Source: CAD feature listing. Evaluate the final solid. Frame: model axes, mm. A direction names the side the tool comes from. Give positions to 0.01 mm unless a question says otherwise; leave off trailing zeros. Order: outer loops, then holes, each group sorted by start corner. A loop starts at its lowest first (then second) coordinate and runs counter-clockwise, first axis right, second up. Notation, with made-up numbers: (62.5, 17.5) -> (103.5, 17.5) arc R21 ccw to (103.5, 56.5) -> close; hole circle Ø8 at (48.25, 39.25). An arc over 180 degrees is marked (long way). Answer in a Markdown table with one row per item.
Autodesk Inventor part; units mm, degrees
ref_plane "YZ Plane" through (0, 0, 0) normal (1, 0, 0) x (0, 1, 0)
ref_plane "XZ Plane" through (0, 0, 0) normal (0, 1, 0) x (-1, 0, 0)
ref_plane "XY Plane" through (0, 0, 0) normal (0, 0, 1) x (1, 0, 0)
sketch "Sketch1" plane through (0, 0, 0) normal (0, 1, 0) x (-1, 0, 0)
  line L0 (0, 0) -> (20, 0)
  line L1 (20, 0) -> (20, -196.3)
  line L2 (20, -196.3) -> (0, -196.3)
  line L3 (0, -196.3) -> (0, 0)
  dimension "d0" = 20
  dimension "d1" = 196.3
extrude "Extrusion1" add sketch "Sketch1" along normal blind 4
sketch "Sketch2" plane through (0, 4, 0) normal (0, 1, 0) x (1, 0, 0)
  line L0 (-20, 0) -> (0, 0)
  line L1 (0, 0) -> (0, 196.3)
  line L2 (-20, 0) -> (0, 0)
  line L3 (0, 0) -> (0, 8)
  line L4 (0, 8) -> (-20, 8)
  line L5 (-20, 8) -> (-20, 0)
  line L6 (-20, 8) -> (0, 8)
  line L7 (0, 8) -> (0, 48.3)
  line L8 (0, 48.3) -> (-20, 48.3)
  line L9 (-20, 48.3) -> (-20, 8)
  line L10 (-20, 48.3) -> (0, 48.3)
  line L11 (0, 48.3) -> (0, 56.3)
  line L12 (0, 56.3) -> (-20, 56.3)
  line L13 (-20, 56.3) -> (-20, 48.3)
  line L14 (-20, 196.3) -> (-20, 0)
  line L15 (-20, 196.3) -> (0, 196.3)
  line L16 (0, 196.3) -> (0, 188.3)
  line L17 (0, 188.3) -> (-20, 188.3)
  line L18 (-20, 188.3) -> (-20, 196.3)
  line L19 (-20, 188.3) -> (0, 188.3)
  line L20 (0, 188.3) -> (0, 148)
  line L21 (0, 148) -> (-20, 148)
  line L22 (-20, 148) -> (-20, 188.3)
  line L23 (-20, 148) -> (0, 148)
  line L24 (0, 148) -> (0, 140)
  line L25 (0, 140) -> (-20, 140)
  line L26 (-20, 140) -> (-20, 148)
  line L27 (-20, 0) -> (-15, 0)
  line L28 (-15, 0) -> (-15, 8)
  line L29 (-15, 8) -> (-20, 8)
  line L30 (-20, 8) -> (-20, 0)
  line L31 (0, 8) -> (-5, 8)
  line L32 (-5, 8) -> (-5, 0)
  line L33 (-5, 0) -> (0, 0)
  line L34 (0, 0) -> (0, 8)
  line L35 (-20, 48.3) -> (-15, 48.3)
  line L36 (-15, 48.3) -> (-15, 56.3)
  line L37 (-15, 56.3) -> (-20, 56.3)
  line L38 (-20, 56.3) -> (-20, 48.3)
  line L39 (0, 48.3) -> (-5, 48.3)
  line L40 (-5, 48.3) -> (-5, 56.3)
  line L41 (-5, 56.3) -> (0, 56.3)
  line L42 (0, 56.3) -> (0, 48.3)
  line L43 (-20, 140) -> (-15, 140)
  line L44 (-15, 140) -> (-15, 148)
  line L45 (-15, 148) -> (-20, 148)
  line L46 (-20, 148) -> (-20, 140)
  line L47 (0, 140) -> (-5, 140)
  line L48 (-5, 140) -> (-5, 148)
  line L49 (-5, 148) -> (0, 148)
  line L50 (0, 148) -> (0, 140)
  line L51 (-20, 188.3) -> (-15, 188.3)
  line L52 (-15, 188.3) -> (-15, 196.3)
  line L53 (-15, 196.3) -> (-20, 196.3)
  line L54 (-20, 196.3) -> (-20, 188.3)
  line L55 (0, 188.3) -> (-5, 188.3)
  line L56 (-5, 188.3) -> (-5, 196.3)
  line L57 (-5, 196.3) -> (0, 196.3)
  line L58 (0, 196.3) -> (0, 188.3)
  point P0 (0, 188.3)
  point P1 (-15, 140)
  point P2 (-20, 148)
  point P3 (-20, 140)
  dimension "d4" = 8
  dimension "d5" = 40.3
  dimension "d6" = 8
  dimension "d7" = 20
  dimension "d8" = 8
  dimension "d9" = 40.3
  dimension "d10" = 8
  dimension "d11" = 5
  dimension "d12" = 5
  dimension "d13" = 8
  dimension "d14" = 5
  dimension "d15" = 5
  dimension "d16" = 5
  dimension "d17" = 5
  dimension "d18" = 5
  dimension "d19" = 5
extrude "Extrusion2" add sketch "Sketch2" along normal blind 10 contours L5 L4 L28 L0 | L32 L4 L1 L0 | L13 L12 L36 L8 | L40 L12 L1 L8 | L14 L21 L44 L25 | L14 L15 L52 L17 | L48 L21 L1 L25 | L56 L15 L1 L17
sketch "Sketch3" plane through (0, 14, 0) normal (0, 1, 0) x (1, 0, 0)
  line L0 (-20, 196.3) -> (-20, 0)
  line L1 (-20, 0) -> (-17.5, 0)
  line L2 (-17.5, 0) -> (-17.5, 4)
  line L3 (-17.5, 4) -> (-20, 4)
  line L4 (-20, 4) -> (-20, 0)
  line L5 (0, 0) -> (0, 196.3)
  line L6 (0, 0) -> (-2.5, 0)
  line L7 (-2.5, 0) -> (-2.5, 4)
  line L8 (-2.5, 4) -> (0, 4)
  line L9 (0, 4) -> (0, 0)
  line L10 (-15, 56.3) -> (-20, 56.3)
  line L11 (-20, 56.3) -> (-17.5, 56.3)
  line L12 (-17.5, 56.3) -> (-17.5, 52.3)
  line L13 (-17.5, 52.3) -> (-20, 52.3)
  line L14 (-20, 52.3) -> (-20, 56.3)
  line L15 (-5, 56.3) -> (0, 56.3)
  line L16 (-5, 56.3) -> (-2.5, 56.3)
  line L17 (-2.5, 56.3) -> (-2.5, 52.3)
  line L18 (-2.5, 52.3) -> (-5, 52.3)
  line L19 (-5, 52.3) -> (-5, 56.3)
  line L20 (-20, 196.3) -> (-17.5, 196.3)
  line L21 (-17.5, 196.3) -> (-17.5, 192.3)
  line L22 (-17.5, 192.3) -> (-20, 192.3)
  line L23 (-20, 192.3) -> (-20, 196.3)
  line L24 (-5, 196.3) -> (-2.5, 196.3)
  line L25 (-2.5, 196.3) -> (-2.5, 192.3)
  line L26 (-2.5, 192.3) -> (-5, 192.3)
  line L27 (-5, 192.3) -> (-5, 196.3)
  line L28 (-20, 148) -> (-15, 148)
  line L29 (-15, 148) -> (-17.5, 148)
  line L30 (-17.5, 148) -> (-17.5, 144)
  line L31 (-17.5, 144) -> (-15, 144)
  line L32 (-15, 144) -> (-15, 148)
  line L33 (-5, 148) -> (-2.5, 148)
  line L34 (-2.5, 148) -> (-2.5, 144)
  line L35 (-2.5, 144) -> (-5, 144)
  line L36 (-5, 144) -> (-5, 148)
  circle A0 centre (-17.5, 144) radius 1.5
  circle A1 centre (-2.5, 144) radius 1.5
  circle A2 centre (-17.5, 192.3) radius 1.5
  circle A3 centre (-2.5, 192.3) radius 1.5
  circle A4 centre (-17.5, 52.3) radius 1.5
  circle A5 centre (-2.5, 52.3) radius 1.5
  circle A6 centre (-17.5, 4) radius 1.5
  circle A7 centre (-2.5, 4) radius 1.5
  dimension "d22" = 2.5
  dimension "d23" = 4
  dimension "d24" = 2.5
  dimension "d25" = 4
  dimension "d26" = 2.5
  dimension "d27" = 4
  dimension "d28" = 2.5
  dimension "d29" = 4
  dimension "d30" = 2.5
  dimension "d31" = 4
  dimension "d32" = 2.5
  dimension "d33" = 4
  dimension "d34" = 2.5
  dimension "d35" = 4
  dimension "d36" = 2.5
  dimension "d37" = 4
  dimension "d38" = 3
  dimension "d39" = 3
  dimension "d40" = 3
  dimension "d41" = 3
  dimension "d42" = 3
  dimension "d43" = 3
  dimension "d44" = 3
  dimension "d45" = 3
extrude "Extrusion3" cut sketch "Sketch3" against normal up to surface (14 mm away) contours A2 L21 L22 | L22 L21 A2 | A0 L31 L30 | L30 L31 A0 | A4 L12 L13 | L13 L12 A4 | A6 L2 L3 | L3 L2 A6 | A7 L7 L8 | L8 L7 A7 | A5 L18 L17 | L17 L18 A5 | A3 L26 L25 | L25 L26 A3 | A1 L35 L34 | L34 L35 A1
fillet "Fillet1" radius 3 12 edges at (-15, 4, -52.3) (-5, 4, -52.3) (-15, 4, -144) (-2.5, 4, -140) (-2.5, 4, -56.3) (-5, 4, -144) (-15, 4, -4) (-5, 4, -4) (-15, 4, -192.3) (-5, 4, -192.3) (-17.5, 4, -56.3) (-17.5, 4, -140)
sketch "Sketch5" plane through (0, 4, 0) normal (0, 1, 0) x (1, 0, 0)
  line L0 (0, 48.3) -> (-8, 48.3)
  line L1 (0, 48.3) -> (-4, 48.3)
  line L2 (-8, 148) -> (0, 148)
  line L3 (0, 148) -> (-4, 148)
  line L4 (-4, 148) -> (-16, 148)
  line L5 (-16, 148) -> (-16, 168)
  line L6 (-16, 168) -> (-4, 168)
  line L7 (-4, 168) -> (-4, 148)
  line L8 (-4, 48.3) -> (-16, 48.3)
  line L9 (-16, 48.3) -> (-16, 28.3)
  line L10 (-16, 28.3) -> (-4, 28.3)
  line L11 (-4, 28.3) -> (-4, 48.3)
  point P0 (0, 0)
  dimension "d63" = 4
  dimension "d64" = 4
  dimension "d65" = 12
  dimension "d66" = 20
  dimension "d67" = 12
  dimension "d68" = 20
extrude "Extrusion5" cut sketch "Sketch5" against normal blind 8
sketch "Sketch6" plane through (0, 0, 0) normal (0, -1, 0) x (1, 0, 0)
  circle A0 centre (-2.5, -4) radius 1.5
  circle A1 centre (-2.5, -4) radius 4
  circle A2 centre (-17.5, -4) radius 1.5
  circle A3 centre (-17.5, -4) radius 4
  circle A4 centre (-17.5, -52.3) radius 1.5
  circle A5 centre (-17.5, -52.3) radius 4
  circle A6 centre (-2.5, -52.3) radius 1.5
  circle A7 centre (-2.5, -52.3) radius 4
  circle A8 centre (-17.5, -144) radius 1.5
  circle A9 centre (-17.5, -144) radius 4
  circle A10 centre (-2.5, -144) radius 1.5
  circle A11 centre (-2.5, -144) radius 4
  circle A12 centre (-17.5, -192.3) radius 1.5
  circle A13 centre (-17.5, -192.3) radius 4
  circle A14 centre (-2.5, -192.3) radius 1.5
  circle A15 centre (-2.5, -192.3) radius 4
  line L0 (0, -196.3) -> (-20, -196.3)
  line L1 (-20, -196.3) -> (-17.5, -196.3)
  line L2 (-17.5, -196.3) -> (-17.5, -192.3)
  line L3 (-17.5, -192.3) -> (-20, -192.3)
  line L4 (-20, -192.3) -> (-20, -196.3)
  line L5 (0, -196.3) -> (-2.5, -196.3)
  line L6 (-2.5, -196.3) -> (-2.5, -192.3)
  line L7 (-2.5, -192.3) -> (0, -192.3)
  line L8 (0, -192.3) -> (0, -196.3)
  line L9 (-20, -196.3) -> (-20, 0)
  line L10 (-20, 0) -> (-17.5, 0)
  line L11 (-17.5, 0) -> (-17.5, -4)
  line L12 (-17.5, -4) -> (-20, -4)
  line L13 (-20, -4) -> (-20, 0)
  line L14 (0, 0) -> (-2.5, 0)
  line L15 (-2.5, 0) -> (-2.5, -4)
  line L16 (-2.5, -4) -> (0, -4)
  line L17 (0, -4) -> (0, 0)
  dimension "d71" = 8
  dimension "d72" = 8
  dimension "d73" = 8
  dimension "d74" = 8
  dimension "d75" = 8
  dimension "d76" = 8
  dimension "d77" = 8
sketch "Sketch7" plane through (0, 4, 0) normal (0, 1, 0) x (1, 0, 0)
  line L0 (-20, 188.3) -> (-20, 148)
  line L1 (-20, 140) -> (-15, 140)
  line L2 (-20, 56.3) -> (-18, 56.3)
  line L3 (-18, 56.3) -> (-18, 140)
  line L4 (-18, 140) -> (-20, 140)
  line L5 (-20, 140) -> (-20, 56.3)
  point P0 (0, 0)
  dimension "d78" = 2
extrude "Extrusion6" add sketch "Sketch7" along normal blind 10
sketch "Sketch8" plane through (0, 4, 0) normal (0, 1, 0) x (1, 0, 0)
  line L0 (0, 59.3) -> (0, 137)
  line L1 (0, 59.3) -> (0, 137)
  line L2 (0, 137) -> (0, 59.3)
  line L3 (0, 0) -> (0, 196.3)
  line L4 (0, 98.15) -> (0, 128.15)
  line L5 (0, 128.15) -> (-2.5, 128.15)
  line L6 (-2.5, 128.15) -> (-2.5, 68.15)
  line L7 (-2.5, 68.15) -> (0, 68.15)
  line L8 (0, 68.15) -> (0, 128.15)
  line L9 (-2.5, 128.15) -> (-12.5, 128.15)
  line L10 (-12.5, 128.15) -> (-12.5, 68.15)
  line L11 (-12.5, 68.15) -> (-2.5, 68.15)
  line L12 (-2.5, 68.15) -> (-2.5, 128.15)
  circle A0 centre (-12.5, 128.15) radius 1.5
  circle A1 centre (-2.5, 128.15) radius 1.5
  circle A2 centre (-12.5, 68.15) radius 1.5
  circle A3 centre (-2.5, 68.15) radius 1.5
  line L13 (-12.5, 128.15) -> (-2.5, 128.15)
  line L14 (-2.5, 128.15) -> (-2.5, 118.15)
  line L15 (-2.5, 118.15) -> (-12.5, 118.15)
  line L16 (-12.5, 118.15) -> (-12.5, 128.15)
  line L17 (-12.5, 68.15) -> (-2.5, 68.15)
  line L18 (-2.5, 68.15) -> (-2.5, 78.15)
  line L19 (-2.5, 78.15) -> (-12.5, 78.15)
  line L20 (-12.5, 78.15) -> (-12.5, 68.15)
  circle A4 centre (-12.5, 118.15) radius 1.5
  circle A5 centre (-2.5, 118.15) radius 1.5
  circle A6 centre (-12.5, 78.15) radius 1.5
  circle A7 centre (-2.5, 78.15) radius 1.5
  dimension "d81" = 30
  dimension "d82" = 2.5
  dimension "d83" = 60
  dimension "d84" = 10
  dimension "d85" = 3
  dimension "d86" = 3
  dimension "d87" = 3
  dimension "d88" = 3
  dimension "d89" = 10
  dimension "d90" = 10
  dimension "d91" = 3
  dimension "d92" = 3
  dimension "d93" = 3
  dimension "d94" = 3
extrude "Extrusion7" cut sketch "Sketch8" against normal blind 10 contours A3 L11 L7 | L7 L6 A3 | L11 A3 L6 | A1 L6 L5 | L5 L9 A1 | A7 L19 L6 | L6 A7 | A2 L10 L11 | L11 L10 A2 | L6 A1 L9 | L19 A7 L6 | A0 L10 L9 | L9 L10 A0 | A5 L6 | L6 L15 A5 | A6 L10 L19 | L19 L10 A6 | A6 L10 | L6 A5 L15 | A4 L15 L10 | L10 A4 | A4 L10 L15
properties part number "support_2_servos"
(1) First-contact query: pin 1 Ø2.5 at (x, z) = (-2.5, -78.15) entering from -Y. Flat tip, straight axial feed; report the tip coordinate or a pass-through.
A:
| item | result |
|---|---|
| pin 1 | passes through |
(2) Pull-direction query (Z, two-part tool) for faces 4 (the cylindrical face through (-5.86, 4.9, -192.36)), 5 (the cylindrical face through (-12.825, 2.028, -126.686)); classes: +Z half, -Z half, draft (parallel to the pull), parting line (faces both ways), or undercut.
A:
| item | result |
|---|---|
| face 4 | draft |
| face 5 | undercut |
(3) Access query for faces 1 (the flat face through (-3, 9, -188.3)), 2 (the cylindrical face through (-3.17, 4.9, -139.14)), 3 (the cylindrical face through (-14.1, 4.86, -143.8)). Directions: +Z, -Z, +X, -X, +Y, -Y. A direction counts if a zero-diameter tool reaches every point of the face in a straight line with its end or side. Return the directions, or none.
A:
| item | result |
|---|---|
| face 1 | +X, -X, +Y |
| face 2 | +X, +Y |
| face 3 | +Z, -Z, +Y |
(4) Ray query, probe 1 along X at (y, z) = (1.3, -78.15); probe 2 along Z at (x, y) = (-5.75, 2.25); probe 3 along X at (y, z) = (3.5, -52.3). Return the intervals inside material, ascending.
A:
| item | result |
|---|---|
| probe 1 | x = -20 to -14, -11 to -4, -1 to 0 |
| probe 2 | z = -196.3 to -168, -148 to -48.3, -28.3 to 0 |
| probe 3 | x = -20 to -19, -16 to -4, -1 to 0 |
(5) Section query A-A (z = -23.5). Return the cut outline in (x, y).
A:
| item | result |
|---|---|
| outline | (-20, 0) -> (0, 0) -> (0, 4) -> (-20, 4) -> close |
